Could you check a few things on this drawing? It's one solid part, dimensions in mm from its lowest x, y, z. A direction names the side the tool comes from. Give positions to 0.01 mm unless a question says otherwise; leave off trailing zeros. Loops run counter-clockwise (first coordinate to the right, second up) from the corner with the lowest first, then second, coordinate; pieces in that order, holes last. Notation, with made-up numbers: M 11,81 L 41,81 A28 ccw 41,113 Z; hole C 77.5,38 d2. An arc over 180 degrees is marked long. Answer as CSV lines item,"result". Start each with the question number.
Item 1: I want a section at D-D on y = 3.75. List the corners of the cut face in (x, z) for me.
Item 2: I want a section at A-A on y = 21. List the corners of the cut face in (x, z) for me (1 decimal).
Item 3: I want a section at B-B on z = 12.5. List the corners of the cut face in (x, y) for me (1 decimal).
Item 4: I want a section at C-C on x = 35.5. List the corners of the cut face in (y, z) for me.
Item 5: If I drill on line 1 along X through (y, z) = (20, 19) (1 decimal); line 2 along Y through (x, z) = (34.5, 17); line 3 along X through (y, z) = (5.75, 5), over which ranges is the centre line in solid material (lowest first)? Write a range as from..to.
Item 6: Will these pins go through, and if not, where does the flat tip stop? P1, Ø3, axis at y = 21.5, z = 16, coming from the +X side; P2, Ø8, axis at y = 23.5, z = 23, coming from the -X side; P3, Ø3, axis at x = 2, z = 23, coming from the +Y side.
Item 7: For the marked faces 1, 2 and 3, which set-ups out of +Z, -Z, +X, -X, +Y, -Y let a thin tool reach every point of the face, with its end or its side?
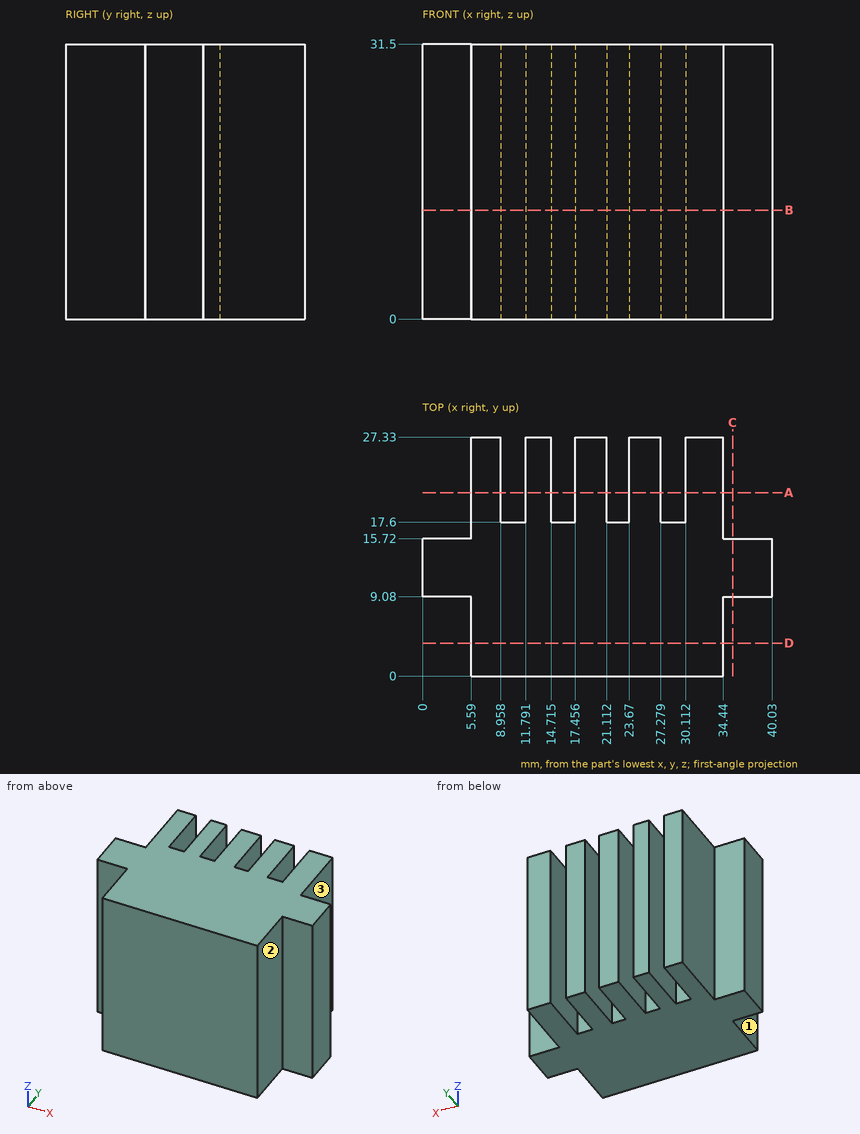
Result:
1,outline,"M 5.59,0 L 34.44,0 L 34.44,31.5 L 5.59,31.5 Z"
2,outline,"M 5.6,0 L 9,0 L 9,31.5 L 5.6,31.5 Z; M 11.8,0 L 14.7,0 L 14.7,31.5 L 11.8,31.5 Z; M 17.5,0 L 21.1,0 L 21.1,31.5 L 17.5,31.5 Z; M 23.7,0 L 27.3,0 L 27.3,31.5 L 23.7,31.5 Z; M 30.1,0 L 34.4,0 L 34.4,31.5 L 30.1,31.5 Z"
3,outline,"M 0,9.1 L 5.6,9.1 L 5.6,0 L 34.4,0 L 34.4,9.1 L 40,9.1 L 40,15.7 L 34.4,15.7 L 34.4,27.3 L 30.1,27.3 L 30.1,17.6 L 27.3,17.6 L 27.3,27.3 L 23.7,27.3 L 23.7,17.6 L 21.1,17.6 L 21.1,27.3 L 17.5,27.3 L 17.5,17.6 L 14.7,17.6 L 14.7,27.3 L 11.8,27.3 L 11.8,17.6 L 9,17.6 L 9,27.3 L 5.6,27.3 L 5.6,15.7 L 0,15.7 Z"
4,outline,"M 9.08,0 L 15.72,0 L 15.72,31.5 L 9.08,31.5 Z"
5,line 1,"5.6..9, 11.8..14.7, 17.5..21.1, 23.7..27.3, 30.1..34.4"
5,line 2,"9.08..15.72"
5,line 3,"5.59..34.44"
6,P1,"x = 34.44"
6,P2,"x = 5.59"
6,P3,"y = 15.72"
7,face 1,"+Z, -Z, -X, -Y"
7,face 2,"+Z, -Z, +X, -Y"
7,face 3,"+Z, -Z, +X, +Y"
